from build123d import *

# Parameters (mm, degrees)
F1_DEPTH = 25.4


with BuildPart() as f1:
    # F0 (on Front) → F1 (new body)
    with BuildSketch(Plane.XZ):
        with BuildLine():
            Line((25.4, 50.8), (0, 50.8))
            Line((0, 50.8), (0, 0))
            Line((0, 0), (50.8, 0))
            Line((50.8, 0), (50.8, 25.4))
            ThreePointArc((50.8, 25.4), (32.839488, 32.839488), (25.4, 50.8))
        make_face()
    extrude(amount=F1_DEPTH)


solid = f1.part
Can you work these out from the model? Positions are in its coordinate system, mm. Coordinates: 2 decimals unless noted, no trailing zeros. Loops run counter-clockwise (first coordinate to the right, second up) from the corner with the lowest first, then second, coordinate; pieces in that order, holes last. Notation, with made-up numbers: (19.5, -16) - (37.5, -16) arc R29 cw to (37.5, 23) - close; hole circle Ø11 at (-1.75, 26.25). An arc over 180 degrees is marked (long way). Answer as a JSON object with one key per item and string values. Group by question number.
Item 1: If we section it at C-C (z = 44): List the corners of the cut face in (x, y) for me.
Item 2: If I drill on L1, parallel to Z at x = 46, y = -7.25; L2, parallel to X at y = -15.75, z = 42; L3, parallel to Z at x = 34, y = -4.5, over which ranges is the centre line in solid material (lowest first)? Write a range as from..to.
Item 3: If we section it at B-B (x = 26.5): List the corners of the cut face in (y, z) for me, plus the area to 3 significant figures.
Item 4: If we section it at A-A (y = -16): List the corners of the cut face in (x, z) for me, plus the area to 3 significant figures.
Item 5: For pin 1 (3 mm diameter, centred on x = 37, y = -4.5, fed in from +Z); pin 2 (1 mm diameter, centred on y = -19.5, z = 30, fed in from +X), each with a flat end and sliding along its axis, tell me the tip position at first contact or that it passes through.
Returned:
{
 "1": {"outline": "(0, -25.4) - (26.33, -25.4) - (26.33, 0) - (0, 0) - close"},
 "2": {"L1": "z = 0..25.86", "L2": "x = 0..26.97", "L3": "z = 0..31.75"},
 "3": {"outline": "(-25.4, 0) - (0, 0) - (0, 43.41) - (-25.4, 43.41) - close", "area": "1,100 mm²"},
 "4": {"outline": "(0, 0) - (50.8, 0) - (50.8, 25.4) arc R25.4 cw to (25.4, 50.8) - (0, 50.8) - close", "area": "2,070 mm²"},
 "5": {"pin 1": "stops at z = 30.53", "pin 2": "stops at x = 36.96"}
}
